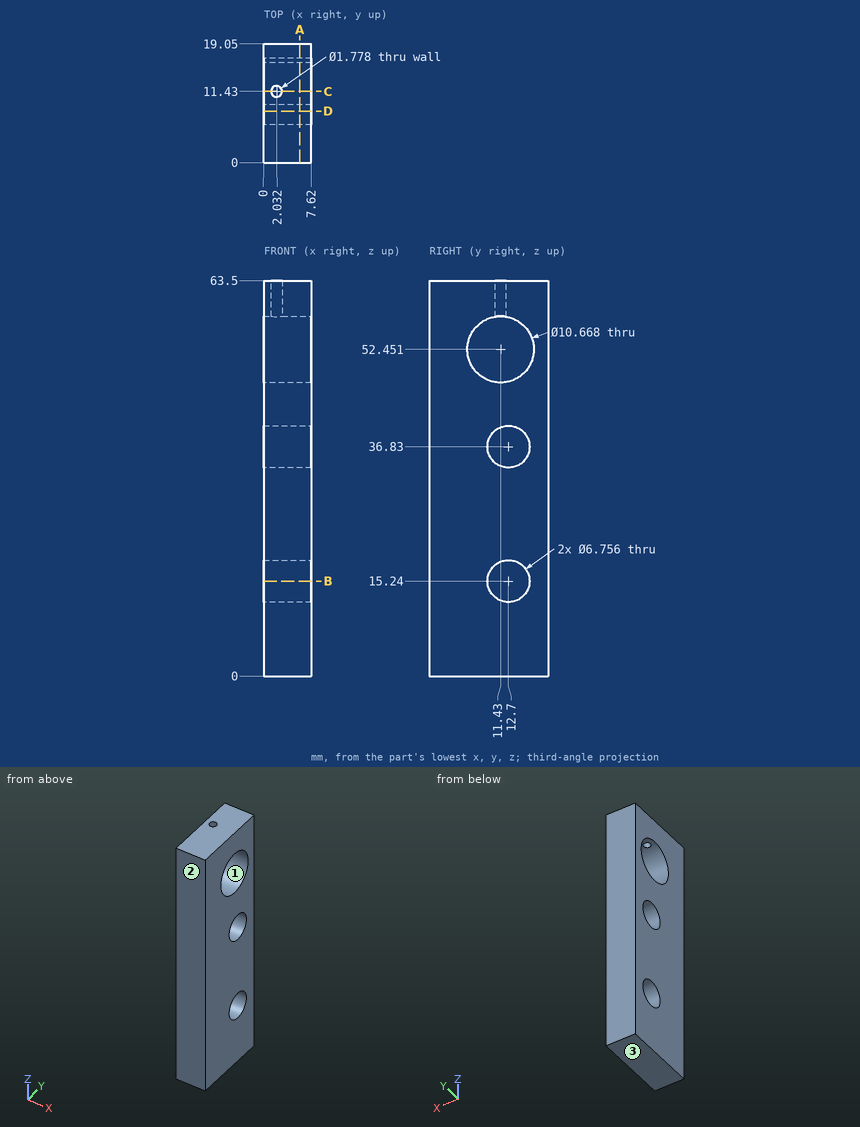
Geometry: see drawing. Coordinates: mm, zero at the bounding-box minimum. Round coordinates to 2 decimals unless told otherwise and drop trailing zeros. Order: outer loops, then holes, each group sorted by start corner. A loop starts at its lowest first (then second) coordinate and runs counter-clockwise, first axis right, second up. Notation, with made-up numbers: (86, 85) -> (144, 85) arc R29 ccw to (144, 106) -> close; hole circle Ø9 at (15.25, 27.5). An arc over 180 degrees is marked (long way). Answer as CSV lines item,"result".
Item 1: Pin query (flat end, axial travel): pin 1 Ø9.5 at (y, z) = (11.43, 52.451) entering from +X; pin 2 Ø2 at (x, y) = (2, 17) entering from -Z. Return the tip coordinate at first contact, or that it passes through.
A:
pin 1,"through"
pin 2,"z = 0"
Item 2: Section D-D, the plane y = 8.25. Return loops of the section in (x, z).
A:
outline,"(0, 0) -> (7.62, 0) -> (7.62, 48.17) -> (0, 48.17) -> close; (0, 56.73) -> (7.62, 56.73) -> (7.62, 63.5) -> (0, 63.5) -> close"
Item 3: Line query: L1, parallel to Y at x = 3.75, z = 15.24; L2, parallel to Y at x = 2.5, z = 52.5; L3, parallel to Z at x = 2, y = 14.75 (1 decimal). Output: solid intervals per line, ascending.
A:
L1,"0 to 9.32, 16.08 to 19.05"
L2,"0 to 6.1, 16.76 to 19.05"
L3,"0 to 12.6, 17.9 to 34.1, 39.5 to 48.3, 56.6 to 63.5"
Item 4: Section C-C, the plane y = 11.43. Return loops of the section in (x, z) (1 decimal), plus the area to 3 significant figures.
A:
outline,"(0, 0) -> (7.6, 0) -> (7.6, 12.1) -> (0, 12.1) -> close; (0, 18.4) -> (7.6, 18.4) -> (7.6, 33.7) -> (0, 33.7) -> close; (0, 40) -> (7.6, 40) -> (7.6, 47.1) -> (0, 47.1) -> close; (0, 57.8) -> (1.1, 57.8) -> (1.1, 63.5) -> (0, 63.5) -> close; (2.9, 57.8) -> (7.6, 57.8) -> (7.6, 63.5) -> (2.9, 63.5) -> close"
area,"297 mm²"
Item 5: Pull-direction query (Z, two-part tool) for the marked faces 1, 2 and 3; classes: pulls with the +Z half, pulls with the -Z half, needs draft (parallel to the pull), parting line crosses it, or undercut.
A:
face 1,"undercut"
face 2,"needs draft"
face 3,"pulls with the -Z half"
Item 6: Section A-A, the plane x = 5.75. Count the separate pieces of the cut face and the enclosed holes in it, plus the area to 3 significant figures.
A:
separate pieces,"1"
enclosed holes,"3"
area,"1,050 mm²"
Item 7: Section B-B, the plane z = 15.24. Return loops of the section in (x, y).
A:
outline,"(0, 0) -> (7.62, 0) -> (7.62, 9.32) -> (0, 9.32) -> close; (0, 16.08) -> (7.62, 16.08) -> (7.62, 19.05) -> (0, 19.05) -> close"
